The listing builds one solid part. Answer for the finished solid, in the listing's coordinates (mm). Give positions to 0.01 mm unless a question says otherwise; leave off trailing zeros. Write each loop counter-clockwise with the first axis right and the second up, starting at its lowest first coordinate (ties: lowest second). Pieces come first, ordered by that corner, then holes. Notation, with made-up numbers: (-39.5, 70) - (12.5, 70) arc R22 cw to (12.5, 89) - close; hole circle Ø6 at (4, 53.5). An arc over 180 degrees is marked (long way). Answer as CSV lines item,"result". Start each with the question number.
(1) For a pull along X with two mould halves and no side action, classify faces 1 (the face through (-38.89, 2.95, 16.08)), 2 (the face through (-31, 40, 316.23)), 3 (the face through (16.3, 20.7, 136.4)), 4 (the face through (-31, 41, 25.4)) as pulls with the +X half, pulls with the -X half, needs draft (parallel to the pull), parting line crosses it, or undercut.
(2) Each of these flat-tipped pins is pushed along its axis until it touches: pin 1 Ø8 at (x, z) = (-55, 83) entering from +Y; pin 2 Ø2 at (y, z) = (7.5, 141) entering from +X; pin 3 Ø8 at (x, z) = (-12.5, 271.5) entering from +Y. Where does it stop, or does it pass through?
(3) Straight lines are drawn through the part: probe 1 along Y at (x, z) = (-60, 17); probe 2 along X at (y, z) = (76.5, 210.5); probe 3 along Z at (x, y) = (5, 29). For each, find the intervals that lie inside material, in ascending order.
(4) Find section A-A (z = 142). Write down the section's boundary in (x, y), then the cut area to 3 significant figures.
from build123d import *

# Parameters (mm, degrees)
F0_R     = 50.8
F1_DEPTH = 311.15
F2_R     = 47.5000066
F3_DEPTH = 5.08
F4_R     = 12.7
F5_DEPTH = 25.4
F6_R     = 5.08


with BuildPart() as f1:
    # F0 (on Top) → F1 (new body)
    with BuildSketch(Plane.XY):
        with Locations((-30.63319996, 40.1448793709)):
            Circle(F0_R)
    extrude(amount=F1_DEPTH)

    # F2
    f2_edges = [f1.edges().sort_by_distance(p)[0] for p in [
        (-81.4332, 40.144879, 311.15),
    ]]
    fillet(f2_edges, radius=F2_R)

    # F3 (add): a face of the model
    f3_faces = [f1.faces().sort_by_distance(p)[0] for p in [
        (-30.63319996, 40.1448793709, 311.15),
    ]]
    extrude(f3_faces, amount=F3_DEPTH)

    # F4
    f4_edges = [f1.edges().sort_by_distance(p)[0] for p in [
        (-81.4332, 40.144879, 0),
    ]]
    fillet(f4_edges, radius=F4_R)

    # F5 (cut): a face of the model
    f5_faces = [f1.faces().sort_by_distance(p)[0] for p in [
        (-30.63319996, 40.1448793709, 0),
    ]]
    extrude(f5_faces, amount=-F5_DEPTH, mode=Mode.SUBTRACT)

    # F6
    f6_edges = [f1.edges().sort_by_distance(p)[0] for p in [
        (-68.7332, 40.144879, 0),
    ]]
    fillet(f6_edges, radius=F6_R)


solid = f1.part
Result set:
1,face 1,"undercut"
1,face 2,"needs draft"
1,face 3,"parting line crosses it"
1,face 4,"undercut"
2,pin 1,"y = 86.68"
2,pin 2,"x = 9.11"
2,pin 3,"y = 88.41"
3,probe 1,"-1.31 to 15.87, 64.42 to 81.6"
3,probe 2,"-66.11 to 4.85"
3,probe 3,"25.4 to 296.78"
4,outline,"circle Ø101.6 at (-30.63, 40.14)"
4,area,"8,110 mm^2"
